Check sheet for the modelled part. Datum: model origin and axes. Units: mm. Coordinates: 2 decimals unless noted, no trailing zeros. Write each question's results on one line, items separated by ' | '. Start each with the question number.
from build123d import *

# Parameters (mm, degrees)
ESQUISSE1_R        = 1.578798566
ESQUISSE1_R_2      = 1.5
ESQUISSE1_R_3      = 1.58210763
BOSS_EXTRU_1_DEPTH = 5
CONG_1_R           = 2


with BuildPart() as part:
    # Esquisse1 → Boss.-Extru.1 (new body)
    with BuildSketch(Plane.XY):
        with BuildLine():
            Line((20.236568094, -45.190021555), (-21.667832927, -39.130000484))
            ThreePointArc((-21.667832927, -39.130000484), (-24.732290594, -37.454232491), (-25.952200511, -34.181478458))
            Line((-25.952200511, -34.181478458), (-25.952200511, 34.181478458))
            ThreePointArc((-25.952200511, 34.181478458), (-24.732290594, 37.454232491), (-21.667832927, 39.130000484))
            Line((-21.667832927, 39.130000484), (20.236568094, 45.190021555))
            ThreePointArc((20.236568094, 45.190021555), (24.224954543, 44.021589613), (25.952200511, 40.241499529))
            Line((25.952200511, 40.241499529), (25.952200511, -40.241499529))
            ThreePointArc((25.952200511, -40.241499529), (24.224954543, -44.021589613), (20.236568094, -45.190021555))
        make_face()
        with Locations((13.054361823, -37.76712052)):
            Circle(ESQUISSE1_R, mode=Mode.SUBTRACT)
        with Locations((-19.786707419, -31.079856582)):
            Circle(ESQUISSE1_R_2, mode=Mode.SUBTRACT)
        with Locations((8.417830834, -17.231443917)):
            Circle(ESQUISSE1_R_2, mode=Mode.SUBTRACT)
        with Locations((-15.15017643, -17.231443917)):
            Circle(ESQUISSE1_R_2, mode=Mode.SUBTRACT)
        with Locations((8.417830834, 17.313551547)):
            Circle(ESQUISSE1_R_3, mode=Mode.SUBTRACT)
        with Locations((-15.15017643, 17.231443917)):
            Circle(ESQUISSE1_R_2, mode=Mode.SUBTRACT)
        with Locations((-19.786707419, 31.079856582)):
            Circle(ESQUISSE1_R_2, mode=Mode.SUBTRACT)
        with Locations((13.054361823, 37.845919086)):
            Circle(ESQUISSE1_R_2, mode=Mode.SUBTRACT)
    extrude(amount=BOSS_EXTRU_1_DEPTH)

    # Congé1
    cong_1_edges = [part.edges().sort_by_distance(p)[0] for p in [
        (-24.732290594, 37.454232491, 5),
        (-25.952200511, 0, 5),
        (-24.732290594, -37.454232491, 5),
        (-0.715632416, -42.16001102, 5),
        (24.224954543, -44.021589613, 5),
        (25.952200511, 0, 5),
        (24.224954543, 44.021589613, 5),
        (-0.715632416, 42.16001102, 5),
    ]]
    fillet(cong_1_edges, radius=CONG_1_R)


solid = part.part
1) Release check for a two-part mould opening along Y. For faces 1 (the cylindrical face through (9.85, -16.78, 2.46)), 2 (the cylindrical face through (-0.341, 41.638, 4.399)), 3 (the flat face through (0, 1, 0)) record: +Y half, -Y half, draft (parallel to the pull), parting line (faces both ways), or undercut.
2) Thickness scan on probe 1 along Y at (x, z) = (-18.5, 4.15); probe 2 along Y at (x, z) = (-15, 1.9); probe 3 along X at (y, z) = (-16, 3). Record the ranges inside material, lowest first.
3) Gauge pin test, flat end, axial feed: P1, Ø3, axis at x = 11.5, z = 1, coming from the -Y side. Record the tip position at first contact, or that the pin passes through.
4) Section check A-A (z = 3.8). Give the number of separate pieces and of enclosed holes in the cut face, then the cut area to 3 significant figures.
Return value:
1) face 1: undercut | face 2: +Y half | face 3: draft
2) probe 1: y = -39.22 to -31.85, -30.31 to 30.31, 31.85 to 39.22 | probe 2: y = -40.09 to -18.72, -15.74 to 15.74, 18.72 to 40.09 | probe 3: x = -25.95 to -16.01, -14.29 to 7.56, 9.27 to 25.95
3) P1: stops at y = -44.14
4) separate pieces: 1 | enclosed holes: 8 | area: 4,260 mm2
